The model under review builds one solid part; all positions refer to its coordinate system, in mm. Face numbers are marked on the shaded views. A direction names the side the tool comes from. Coordinates: 2 decimals unless noted, no trailing zeros. Write each loop counter-clockwise with the first axis right and the second up, starting at its lowest first coordinate (ties: lowest second). Pieces come first, ordered by that corner, then holes. Notation, with made-up numbers: (88.5, -39) - (114.5, -39) arc R19 cw to (114.5, -25) - close; hole circle Ø4 at (-40, 28). An arc over 180 degrees is marked (long way). Use one line per item in the form item = value. Start each with the question number.
```python
from build123d import *

# Parameters (mm, degrees)
PAD_DEPTH = 40


with BuildPart() as part:
    # Sketch → Pad (new body)
    with BuildSketch(Plane.XY):
        Polygon((0, 0), (20, 0), (20, -50), (25, -50), (25, 5), (10, 5), (10, 35), (0, 35), align=None)
    pad = extrude(amount=PAD_DEPTH)

    # Mirrored: Pad across Sketch V_Axis
    add(pad.mirror(Plane(origin=(0, 0, 0), x_dir=(0, 0, 1), z_dir=(1, 0, 0))))


solid = part.part
```
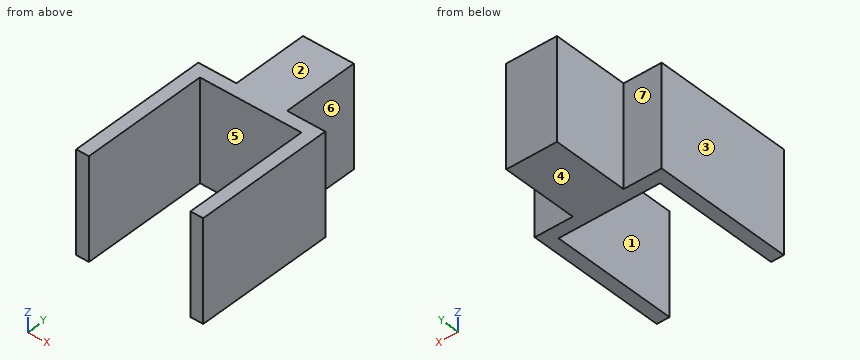
1. For P1, Ø9, axis at y = 19, z = 23, coming from the -X side; P2, Ø3, axis at x = 12.5, y = 9, coming from the -Z side; P3, Ø12, axis at x = -14.5, z = 17.5, coming from the +Y side; P4, Ø1, axis at x = 16.5, z = 8, coming from the -Y side, all flat-tipped, find the tip position at first contact; note any pin that passes through.
2. Take a section at C-C (x = -11.5). State the section outline as (y, z) points.
3. For L1, parallel to X at y = -14, z = 30; L2, parallel to X at y = 16, z = 37; L3, parallel to Y at x = -13.5, z = 3, list the stretches that pass through material, from the lowest coordinate up.
4. The part is to be moulded in two halves that separate along X. For the marked faces 1, 2 and 3, say which applies: released by +X, released by -X, zero draft, split by the parting line, or undercut.
5. Take a section at A-A (y = -21). State the section outline as (x, z) points.
6. For the marked faces 4, 5, 6 and 7, list the 3-axis set-ups (+Z, -Z, +X, -X, +Y, -Y) from which the entire face can be reached by the end or side of a thin tool; tool diameter is ignored.
7. Take a section at B-B (z = 34). State the section outline as (x, y) points.
8. Take a section at D-D (y = 17). State the section outline as (x, z) points, plus the area to 3 significant figures.
Returned:
q1.P1 = -10
q1.P2 = through
q1.P3 = 35
q1.P4 = 0
q2.outline = (0, 0) - (5, 0) - (5, 40) - (0, 40) - close
q3.L1 = -25 to -20, 20 to 25
q3.L2 = -10 to 10
q3.L3 = 0 to 5
q4.face_1 = undercut
q4.face_2 = zero draft
q4.face_3 = released by -X
q5.outline = (-25, 0) - (-20, 0) - (-20, 40) - (-25, 40) - close; (20, 0) - (25, 0) - (25, 40) - (20, 40) - close
q6.face_4 = -Z, +X, -X, +Y, -Y
q6.face_5 = +Z, -Z, -Y
q6.face_6 = +Z, -Z, +X, +Y
q6.face_7 = +Z, -Z, -X, +Y
q7.outline = (-25, -50) - (-20, -50) - (-20, 0) - (20, 0) - (20, -50) - (25, -50) - (25, 5) - (10, 5) - (10, 35) - (-10, 35) - (-10, 5) - (-25, 5) - close
q8.outline = (-10, 0) - (10, 0) - (10, 40) - (-10, 40) - close
q8.area = 800 mm²
